from build123d import *

# Parameters (mm, degrees)
F0_R     = 7.14375
F0_R_2   = 33.3375
F0_R_3   = 8.509
F0_R_4   = 8.89
F1_DEPTH = 6.35


# Not quite as in the source:
# - ends of sketch curves that miss each other by under 0.0002 mm in the source are joined


with BuildPart() as f1:
    # F0 (on Front) → F1 (new body)
    with BuildSketch(Plane.XZ):
        with BuildLine():
            Line((-990.675184, -31.5729874), (-1041.475184, -31.5729874))
            Line((-1041.475184, -31.5729874), (-1041.475184, -374.4729874))
            ThreePointArc((-1041.475184, -374.4729874), (-1039.6153120605, -378.9631154605), (-1035.125184, -380.8229874))
            Line((-1035.125184, -380.8229874), (888.924816, -380.8229874))
            ThreePointArc((888.924816, -380.8229874), (893.4149440605, -378.9631154605), (895.274816, -374.4729874))
            Line((895.274816, -374.4729874), (895.274816, -317.3229874))
            ThreePointArc((895.274816, -317.3229874), (910.1537915157, -281.4019629157), (946.074816, -266.5229874))
            Line((946.074816, -266.5229874), (1041.4752094, -266.5229874))
            Line((1041.4752094, -266.5229874), (1041.4752094, 19.626326))
            Line((1041.4752094, 19.626326), (611.3003013693, 73.7272843556))
            ThreePointArc((611.3003013693, 73.7272843556), (551.322654557, 105.4521002182), (527.3308478102, 168.920007602))
            ThreePointArc((527.3308478102, 168.920007602), (527.3308670888, 168.9390000629), (527.3308558827, 168.9579925234))
            ThreePointArc((527.3308558827, 168.9579925234), (439.9522285654, 340.3269099665), (249.9729787047, 370.4966796024))
            Line((249.9729787047, 370.4966796024), (-990.675184, -31.5729874))
        make_face()
        with Locations((-889.0246634, -266.991084)):
            Circle(F0_R, mode=Mode.SUBTRACT)
        with Locations((-736.6246634, -266.991084)):
            Circle(F0_R, mode=Mode.SUBTRACT)
        with Locations((-635.069342, -266.9311654)):
            Circle(F0_R, mode=Mode.SUBTRACT)
        with Locations((-465.2920082, -266.8996694)):
            Circle(F0_R, mode=Mode.SUBTRACT)
        with Locations((-312.8920082, -266.8996694)):
            Circle(F0_R, mode=Mode.SUBTRACT)
        with Locations((-465.010881, -192.5398994)):
            Circle(F0_R, mode=Mode.SUBTRACT)
        with Locations((-312.610881, -192.5398994)):
            Circle(F0_R, mode=Mode.SUBTRACT)
        with Locations((-160.4920082, -266.8996694)):
            Circle(F0_R, mode=Mode.SUBTRACT)
        with Locations((-8.0920082, -266.8996694)):
            Circle(F0_R, mode=Mode.SUBTRACT)
        with Locations((-46.3986626, -193.1547064)):
            Circle(F0_R, mode=Mode.SUBTRACT)
        with Locations((-888.8878082, -186.200796)):
            Circle(F0_R, mode=Mode.SUBTRACT)
        with Locations((-685.8404368, -173.2472278)):
            Circle(F0_R, mode=Mode.SUBTRACT)
        with Locations((-736.5858268, -89.1617978)):
            Circle(F0_R, mode=Mode.SUBTRACT)
        with Locations((-635.0111506, -89.2015996)):
            Circle(F0_R, mode=Mode.SUBTRACT)
        with Locations((144.3079918, -266.8996694)):
            Circle(F0_R, mode=Mode.SUBTRACT)
        with Locations((163.915471, -193.1547064)):
            Circle(F0_R, mode=Mode.SUBTRACT)
        with Locations((296.7079918, -266.8996694)):
            Circle(F0_R, mode=Mode.SUBTRACT)
        with Locations((434.869844, -266.86002)):
            Circle(F0_R, mode=Mode.SUBTRACT)
        with Locations((714.3297118, -266.927076)):
            Circle(F0_R, mode=Mode.SUBTRACT)
        with Locations((881.4062128, -267.5829294)):
            Circle(F0_R, mode=Mode.SUBTRACT)
        with Locations((965.0764544, -247.1495184)):
            Circle(F0_R, mode=Mode.SUBTRACT)
        with Locations((279.9671566, -89.1229866)):
            Circle(F0_R, mode=Mode.SUBTRACT)
        with Locations((434.915945, -89.109677)):
            Circle(F0_R, mode=Mode.SUBTRACT)
        with Locations((523.8131764, -173.234477)):
            Circle(F0_R, mode=Mode.SUBTRACT)
        with Locations((625.4303722, -173.2491836)):
            Circle(F0_R, mode=Mode.SUBTRACT)
        with Locations((714.2706314, -89.1516632)):
            Circle(F0_R, mode=Mode.SUBTRACT)
        with Locations((-398.852898, 17.0261788)):
            Circle(F0_R, mode=Mode.SUBTRACT)
        with Locations((-335.9403238, 17.0261788)):
            Circle(F0_R_2, mode=Mode.SUBTRACT)
        with Locations((-273.027775, 17.0261788)):
            Circle(F0_R, mode=Mode.SUBTRACT)
        with Locations((-160.4810608, 17.0261788)):
            Circle(F0_R, mode=Mode.SUBTRACT)
        with Locations((-46.3986626, 17.0261788)):
            Circle(F0_R, mode=Mode.SUBTRACT)
        with Locations((-160.4982312, 194.9087288)):
            Circle(F0_R, mode=Mode.SUBTRACT)
        with Locations((7.547102, 17.0261788)):
            Circle(F0_R, mode=Mode.SUBTRACT)
        with Locations((70.4596762, 17.0261788)):
            Circle(F0_R_2, mode=Mode.SUBTRACT)
        with Locations((133.372225, 17.0261788)):
            Circle(F0_R, mode=Mode.SUBTRACT)
        with Locations((200.8515922, 54.1913826)):
            Circle(F0_R_3, mode=Mode.SUBTRACT)
        with Locations((315.8054136, 6.5158112)):
            Circle(F0_R_3, mode=Mode.SUBTRACT)
        with Locations((429.82642, 54.206775)):
            Circle(F0_R_3, mode=Mode.SUBTRACT)
        with Locations((57.5594988, 133.1437774)):
            Circle(F0_R, mode=Mode.SUBTRACT)
        with Locations((153.3248902, 168.9963346)):
            Circle(F0_R_3, mode=Mode.SUBTRACT)
        with Locations((478.0577434, 168.9963346)):
            Circle(F0_R_3, mode=Mode.SUBTRACT)
        with Locations((200.7754176, 283.379291)):
            Circle(F0_R_4, mode=Mode.SUBTRACT)
        with Locations((429.929163, 283.4136826)):
            Circle(F0_R_3, mode=Mode.SUBTRACT)
        with Locations((315.7209586, 331.3233658)):
            Circle(F0_R_3, mode=Mode.SUBTRACT)
    extrude(amount=F1_DEPTH)


solid = f1.part
Model file for the job. Use its own axes, mm. Round coordinates to 2 decimals unless told otherwise and drop trailing zeros. Loops run counter-clockwise (first coordinate to the right, second up) from the corner with the lowest first, then second, coordinate; pieces in that order, holes last.
1. Wall check: probe 1 along X at (y, z) = (-5.5, -89); probe 2 along Z at (x, y) = (-316, -2.75); probe 3 along Z at (x, y) = (-275, -4.5). Give the ranges that are in metal, low to high.
Check values:
probe 1: x = -1041.48 to -743.73, -729.44 to -642.15, -627.87 to 272.82, 287.11 to 427.77, 442.06 to 707.13, 721.41 to 1041.48
probe 2: z = -380.82 to -273.33, -260.47 to -198.83, -186.25 to -9.69, 43.74 to 187.08
probe 3: z = -380.82 to 10.16, 23.89 to 200.36
2. Drop flat-ended pins along their axis: P1, Ø13, axis at x = -465.29, z = -266.9, coming from the -Y side; P2, Ø3, axis at x = -1021, y = -4.5, coming from the +Z side; P3, Ø3, axis at y = -3, z = -336, coming from the +X side. Give the stop position or say it passes through.
Check values:
P1: passes through
P2: stops at z = -31.57
P3: stops at x = 895.27
3. Band-saw the part on A-A, the plane y = -1. Count the separate pieces of the cut face and the enclosed holes in it, and give its area (3 significant figures).
Check values:
separate pieces: 1
enclosed holes: 44
area: 1,100,000 mm2
4. Band-saw the part on B-B, the plane x = -213.5. List the corners of the cut face in (y, z), and give its area (3 significant figures).
Check values:
outline: (-6.35, -380.82) - (0, -380.82) - (0, 220.29) - (-6.35, 220.29) - close
area: 3,820 mm2
5. Band-saw the part on C-C, the plane x = -537. List the corners of the cut face in (y, z), and give its area (3 significant figures).
Check values:
outline: (-6.35, -380.82) - (0, -380.82) - (0, 115.45) - (-6.35, 115.45) - close
area: 3,150 mm2
6. Mould opens along X. For faces 1 (the cylindrical face through (45.89, -3.13, 39.56)), 2 (the cylindrical face through (442.2, -3.13, 338.67)), 3 (the cylindrical face through (551.969, -3.131, 104.727)) say: +X half, -X half, draft (parallel to the pull), parting line (faces both ways), or undercut.
Check values:
face 1: undercut
face 2: parting line
face 3: +X half
